```python
from build123d import *

# Parameters (mm, degrees)
F1_DEPTH = 6.35


with BuildPart() as f1:
    # F0 (on Front) → F1 (new body)
    with BuildSketch(Plane.XZ):
        with BuildLine():
            Line((3.175, -82.55), (38.1, -82.55))
            ThreePointArc((38.1, -82.55), (44.835192, -79.760192), (47.625, -73.025))
            Line((47.625, -73.025), (47.625, 60.325))
            ThreePointArc((47.625, 60.325), (41.115448, 76.040448), (25.4, 82.55))
            Line((25.4, 82.55), (3.175, 82.55))
            Line((3.175, 82.55), (-2.881412, 82.55))
            Line((-2.881412, 82.55), (-25.4, 82.55))
            ThreePointArc((-25.4, 82.55), (-41.115448, 76.040448), (-47.625, 60.325))
            Line((-47.625, 60.325), (-47.625, -73.025))
            ThreePointArc((-47.625, -73.025), (-44.835192, -79.760192), (-38.1, -82.55))
            Line((-38.1, -82.55), (-2.881412, -82.55))
            Line((-2.881412, -82.55), (-2.881412, 1.333451))
            Line((-2.881412, 1.333451), (3.175, 1.3208))
            Line((3.175, 1.3208), (3.175, -82.55))
        make_face()
    extrude(amount=F1_DEPTH)


solid = f1.part
```
Design review of the part built by this model. Coordinates are the model's own, in mm. A direction names the side the tool comes from. Give positions to 0.01 mm unless a question says otherwise; leave off trailing zeros. Order: outer loops, then holes, each group sorted by start corner. A loop starts at its lowest first (then second) coordinate and runs counter-clockwise, first axis right, second up. Notation, with made-up numbers: (-8, -2.75) -> (4, -2.75) arc R20 ccw to (4, 21.25) -> close; hole circle Ø2 at (-12, 44). An arc over 180 degrees is marked (long way). Write item = value, one per line. Start each with the question number.
(1) We need section B-B on y = -4.25. Write out the cut boundary in (x, z) (3 decimals), plus the area to 3 significant figures.
(2) We need section A-A on z = -63.5. Write out the cut boundary in (x, y) (3 decimals).
(3) To check wall thickness, follow line 1 along X through (y, z) = (-2.5, -58) (3 decimals); line 2 along X through (y, z) = (-4.75, -76) (3 decimals); line 3 along Z through (x, y) = (-39, -3.25). State the ranges of each line that lie inside material, in increasing order.
(4) Mouldability with a two-part tool opening along X and no side actions: class faces 1 (the face through (47.625, -3, -7)), 2 (the face through (3.175, -3, -40)), 3 (the face through (0, -3, 82.55)) as +X half, -X half, draft (parallel to the pull), parting line (faces both ways), or undercut.
(5) For pin 1 (1 mm diameter, centred on x = 1.5, z = 23.5, fed in from +Y), flat-tipped, find the tip position at first contact; note if it passes through.
(6) For faces 4 (the face through (-2.881, -3, -41)), 5 (the face through (-21, -3, -82.55)), list the 3-axis set-ups (+Z, -Z, +X, -X, +Y, -Y) from which the entire face can be reached by the end or side of a thin tool; tool diameter is ignored.
Numbers:
q1.outline = (-47.625, -73.025) arc R9.525 ccw to (-38.1, -82.55) -> (-2.881, -82.55) -> (-2.881, 1.333) -> (3.175, 1.321) -> (3.175, -82.55) -> (38.1, -82.55) arc R9.525 ccw to (47.625, -73.025) -> (47.625, 60.325) arc R22.225 ccw to (25.4, 82.55) -> (-25.4, 82.55) arc R22.225 ccw to (-47.625, 60.325) -> close
q1.area = 15,000 mm^2
q2.outline = (-47.625, -6.35) -> (-2.881, -6.35) -> (-2.881, 0) -> (-47.625, 0) -> close; (3.175, -6.35) -> (47.625, -6.35) -> (47.625, 0) -> (3.175, 0) -> close
q3.line_1 = -47.625 to -2.881, 3.175 to 47.625
q3.line_2 = -47.148 to -2.881, 3.175 to 47.148
q3.line_3 = -82.51 to 77.9
q4.face_1 = +X half
q4.face_2 = undercut
q4.face_3 = draft
q5.pin_1 = 0
q6.face_4 = -Z, +Y, -Y
q6.face_5 = -Z, +X, -X, +Y, -Y
